Here's how the part is built. I have some questions about the finished solid (model axes, mm). A direction names the side the tool comes from. Give positions to 0.01 mm unless a question says otherwise; leave off trailing zeros. Loops run counter-clockwise (first coordinate to the right, second up) from the corner with the lowest first, then second, coordinate; pieces in that order, holes last. Notation, with made-up numbers: (42.5, 26) -> (96.5, 26) arc R25 ccw to (96.5, 56) -> close; hole circle Ø9 at (-9.5, 61.5). An arc over 180 degrees is marked (long way). Answer in a Markdown table with one row per item. Add a question column.
Item 1: If I drill on line 1 (X direction, y = 0.7, z = 0); line 2 (Z direction, x = -0.5, y = -7); line 3 (X direction, y = -9, z = 39.5), over which ranges is the centre line in solid material (lowest first)?
Item 2: Which directions (+Z, -Z, +X, -X, +Y, -Y) give clear straight access to the entire face, cutting with the end or side of a thin tool? Please do faces 4 (the face through (-18, -1.418, -50)), 5 (the face through (37.3, 3.582, -37.3)), 6 (the face through (-42.594, -51.884, -55.55)), 7 (the face through (-71, -42.418, 0)), 8 (the face through (-78.1, -45.38, -17.34)).
Item 3: For P1, Ø3, axis at x = -40.66, z = 40.66, coming from the +Y side; P2, Ø4, axis at y = -22, z = -54, coming from the +X side; P3, Ø2, axis at y = -37.5, z = 30.5, coming from the +X side; P4, Ø2, axis at x = -57, z = 42, coming from the +Y side, each with a flat end and sliding along its axis, tell me the tip position at first contact or that it passes through.
Item 4: If we section it at A-A (y = -22.5): Write out the boundary of the cut face in (x, z).
Item 5: We'd pull the mould along Y, two halves only. Please class faces 1 (the face through (-64, -61.418, -18)), 2 (the face through (-70, -49.418, -6)), 3 (the face through (-15.77, 1.046, 50.076)): released by +Y, released by -Y, zero draft, split by the parting line, or undercut.
Solid Edge part; units mm, degrees
sketch "Sketch1" plane through (0, 0, 0) normal (1, 0, 0) x (0, 1, 0)
  line L0 (-42.4185, 70) -> (-3.9185, 70)
  line L1 (3.5815, 62.5) -> (-3.9185, 70)
  line L2 (3.5815, 62.5) -> (3.5815, 52.5)
  line L3 (3.5815, 52.5) -> (-1.4185, 52.5)
  line L4 (-1.4185, 60.4289) -> (-1.4185, 52.5)
  line L5 (-1.4185, 60.4289) -> (-5.9895, 65)
  line L6 (-5.9895, 65) -> (-61.4185, 65)
  line L7 (-61.4185, 80) -> (-61.4185, 65)
  line L8 (-61.4185, 80) -> (-54.4185, 80)
  line L9 (-54.4185, 80) -> (-54.4185, 70)
  line L10 (-54.4185, 70) -> (-49.4185, 70)
  line L11 (-49.4185, 70) -> (-49.4185, 80)
  line L12 (-49.4185, 80) -> (-42.4185, 80)
  line L13 (-42.4185, 80) -> (-42.4185, 70)
  dimension "D1" = 54.4185
  dimension "D2" = 49.4185
  dimension "D3" = 54.4185
  dimension "D4" = 1.4185
revolve "RevolvedProtrusion1" add sketch "Sketch1" angle 360 about axis through (0, -60, 0) along (0, 1, 0)
hole "Bohrung_1" at (0, 3.5815, 57.5) direction (0, -1, 0) diameter 2.459 end up to next
pattern_circular "Pattern1" count 32 over 360 about axis through (0, 3.5815, 0) along (0, -1, 0) of "Bohrung_1"
chamfer "Chamfer1" distance 1 angle 45 2 edges at (0, -49.4185, 80) (0, -54.4185, 80)
chamfer "Fase_3" distance 1 angle 45 1 edges at (0, -61.4185, 65)
chamfer "Fase_4" distance 1 angle 45 1 edges at (0, -61.4185, 80)
properties material "Aluminium Legierung:3.1355 ,  AlCu4Mg1, EN-AW 2024"
Recorded:
| question | item | result |
|---|---|---|
| 1 | line 1 | x = -65.38 to -58.73, -56.27 to -52.5, 52.5 to 56.27, 58.73 to 65.38 |
| 1 | line 2 | z = -70 to -65, 65 to 70 |
| 1 | line 3 | x = -57.79 to -51.62, 51.62 to 57.79 |
| 2 | face 4 | -Y |
| 2 | face 5 | +Z, -Z, +X, -X, +Y |
| 2 | face 6 | none |
| 2 | face 7 | +Y |
| 2 | face 8 | +Y, -Y |
| 3 | P1 | stops at y = 3.58 |
| 3 | P2 | stops at x = 46.86 |
| 3 | P3 | stops at x = 63.48 |
| 3 | P4 | stops at y = -3.72 |
| 4 | outline | circle Ø140 at (0, 0); hole circle Ø130 at (0, 0) |
| 5 | face 1 | released by -Y |
| 5 | face 2 | undercut |
| 5 | face 3 | zero draft |
